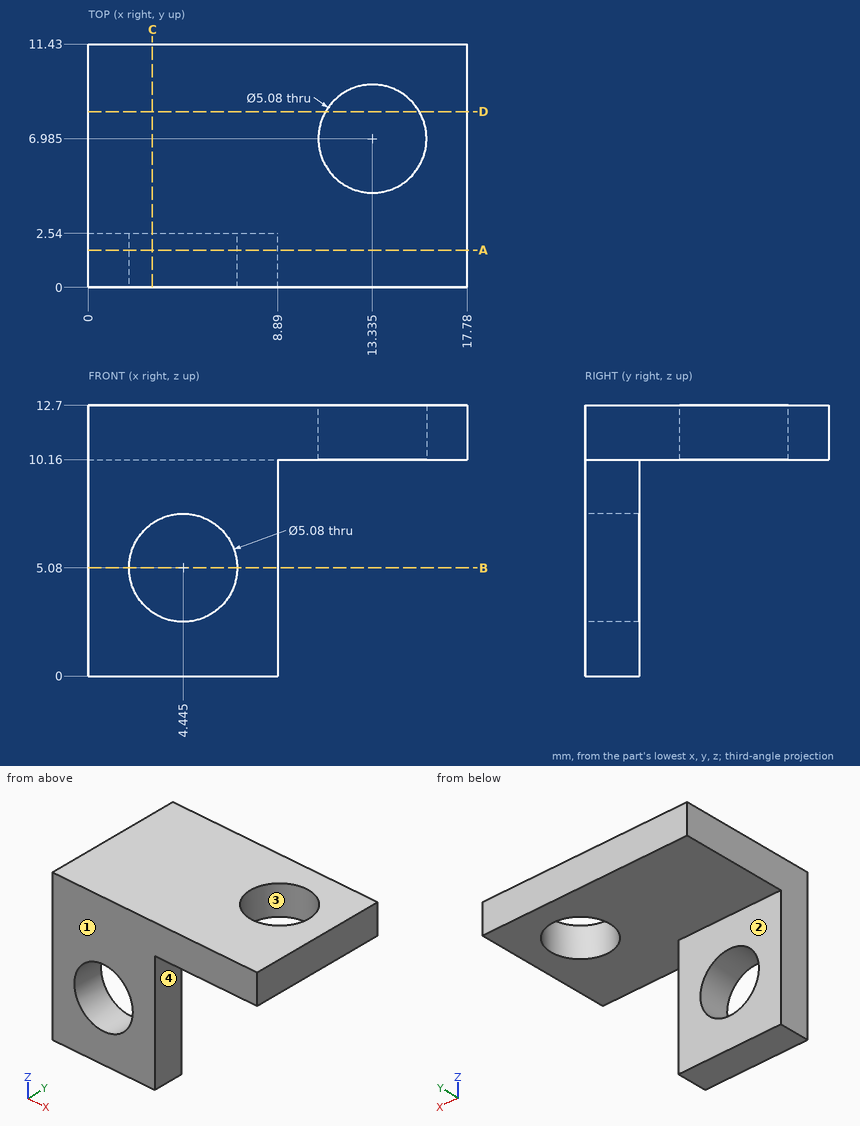
Part print with two shaded views. Sizes in mm from the minimum x, y, z corner. Round coordinates to 2 decimals unless told otherwise and drop trailing zeros. Write each loop counter-clockwise with the first axis right and the second up, starting at its lowest first coordinate (ties: lowest second). Pieces come first, ordered by that corner, then holes. Notation, with made-up numbers: (80.5, 2) - (94.5, 2) arc R15 ccw to (94.5, 22) - close; hole circle Ø5 at (55.5, 40.25). An arc over 180 degrees is marked (long way). Use CSV: the item, a comma, the result in double quotes.
Item 1: Slice it at D-D, the plane y = 8.25. Write the cut outline in (x, z), then the cut area to 3 significant figures.
Results list:
outline,"(0, 10.16) - (11.13, 10.16) - (11.13, 12.7) - (0, 12.7) - close; (15.54, 10.16) - (17.78, 10.16) - (17.78, 12.7) - (15.54, 12.7) - close"
area,"34.0 mm²"
Item 2: Slice it at A-A, the plane y = 1.75. Write the cut outline in (x, z) (3 decimals), then the cut area to 3 significant figures.
Results list:
outline,"(0, 0) - (8.89, 0) - (8.89, 10.16) - (17.78, 10.16) - (17.78, 12.7) - (0, 12.7) - close; hole circle Ø5.08 at (4.445, 5.08)"
area,"115 mm²"
Item 3: Slice it at B-B, the plane z = 5.08. Write the cut outline in (x, y) (3 decimals), then the cut area to 3 significant figures.
Results list:
outline,"(0, 0) - (1.905, 0) - (1.905, 2.54) - (0, 2.54) - close; (6.985, 0) - (8.89, 0) - (8.89, 2.54) - (6.985, 2.54) - close"
area,"9.68 mm²"
Item 4: Slice it at C-C, the plane x = 3. Write the cut outline in (y, z), then the cut area to 3 significant figures.
Results list:
outline,"(0, 0) - (2.54, 0) - (2.54, 2.99) - (0, 2.99) - close; (0, 7.17) - (2.54, 7.17) - (2.54, 10.16) - (11.43, 10.16) - (11.43, 12.7) - (0, 12.7) - close"
area,"44.2 mm²"
Item 5: Pull direction Y, two halves, no side cores. Call the marked faces 1, 2, 3 and 4: pulls with the +Y half, pulls with the -Y half, needs draft (parallel to the pull), parting line crosses it, or undercut.
Results list:
face 1,"pulls with the -Y half"
face 2,"pulls with the +Y half"
face 3,"undercut"
face 4,"needs draft"
Item 6: Wall check: L1, parallel to X at y = 1.4, z = 5.08 (3 decimals); L2, parallel to X at y = 6, z = 10.5; L3, parallel to Z at x = 11, y = 4.5. Give the ranges that are in metal, low to high.
Results list:
L1,"x = 0 to 1.905, 6.985 to 8.89"
L2,"x = 0 to 10.99, 15.68 to 17.78"
L3,"z = 10.16 to 12.7"
Item 7: Flat gauge pins, fed straight in: P1, Ø1, axis at y = 1, z = 3.5, coming from the +X side; P2, Ø2, axis at x = 10.5, z = 6.5, coming from the -Y side; P3, Ø1, axis at x = 2, y = 3.5, coming from the -Z side; P4, Ø2.5, axis at x = 2.5, z = 4, coming from the +Y side. Where does each tip first touch, or does it go through?
Results list:
P1,"stops at x = 8.89"
P2,"passes through"
P3,"stops at z = 10.16"
P4,"stops at y = 2.54"
